```python
from build123d import *

# Parameters (mm, degrees)
SKETCH_1_R          = 4.85
EXTRUDE_1_DEPTH     = 0.5
SKETCH_2_R          = 4
EXTRUDE_2_DEPTH     = 2
SKETCH_3_R          = 3
CUT_EXTRUDE_3_DEPTH = 8.300342458
CHAMFER_1_SIZE      = 0.25


with BuildPart() as part:
    # 草圖1 → 伸長1 (new body)
    with BuildSketch(Plane.XY):
        Circle(SKETCH_1_R)
    extrude(amount=EXTRUDE_1_DEPTH)

    # 草圖2 → 伸長2 (add)
    with BuildSketch(Plane.XY.offset(0.5)):
        Circle(SKETCH_2_R)
    extrude(amount=EXTRUDE_2_DEPTH)

    # 草圖3 → 伸長3 (cut, through all)
    with BuildSketch(Plane.XY.offset(2.5)):
        Circle(SKETCH_3_R)
    extrude(amount=-CUT_EXTRUDE_3_DEPTH, mode=Mode.SUBTRACT)

    # 導角1
    chamfer_1_edges = [part.edges().sort_by_distance(p)[0] for p in [
        (-3, 0, 2.5),
        (-4, 0, 2.5),
    ]]
    chamfer(chamfer_1_edges, length=CHAMFER_1_SIZE)


solid = part.part
```
Verification items for the finished model (mm, model axes). A direction names the side the tool comes from. Round coordinates to 2 decimals unless told otherwise and drop trailing zeros. Loops run counter-clockwise (first coordinate to the right, second up) from the corner with the lowest first, then second, coordinate; pieces in that order, holes last. Notation, with made-up numbers: (75, 29) -> (90, 29) arc R21 ccw to (90, 65) -> close; hole circle Ø11 at (80.25, -22.75). An arc over 180 degrees is marked (long way). Answer as a JSON object with one key per item and string values.
Q1. Access from +Z, -Z, +X, -X, +Y, -Y to the whole of each face (thin tool, end or side, straight path). Record for faces 1 (the flat face through (-1.4, 3.1, 2.5)), 2 (the flat face through (-2, 4, 0.5)).
Data:
{"face 1": "+Z, +X, -X, +Y, -Y", "face 2": "+Z"}
Q2. Section check A-A (y = 0). Record the boundary of the cut face in (x, z), then the cut area to 4 significant figures.
Data:
{"outline": "(-4.85, 0) -> (-3, 0) -> (-3, 2.25) -> (-3.25, 2.5) -> (-3.75, 2.5) -> (-4, 2.25) -> (-4, 0.5) -> (-4.85, 0.5) -> close; (3, 0) -> (4.85, 0) -> (4.85, 0.5) -> (4, 0.5) -> (4, 2.25) -> (3.75, 2.5) -> (3.25, 2.5) -> (3, 2.25) -> close", "area": "5.725 mm2"}
Q3. Draft check along X on faces 3 (the cylindrical face through (-3, 0, 1)), 4 (the flat face through (3.2, 0.1, 0)), 5 (the cylindrical face through (-0.867, -3.905, 1.363)). Enter one of: pulls with the +X half, pulls with the -X half, needs draft (parallel to the pull), parting line crosses it, or undercut.
Data:
{"face 3": "undercut", "face 4": "needs draft", "face 5": "parting line crosses it"}
Q4. Go/stop test with a flat-tipped pin: P1, Ø1.5, axis at y = 1, z = 2, coming from the -X side. Record where the tip stops, or that it passes through.
Data:
{"P1": "stops at x = -3.99"}
Q5. Scan lines: line 1 (Y direction, x = 0, z = 0.9); line 2 (Y direction, x = -0.75, z = 1); line 3 (X direction, y = 1.25, z = 1.1). Record each from-to range of solid material in increasing order. Write a range as from..to.
Data:
{"line 1": "y = -4..-3, 3..4", "line 2": "y = -3.93..-2.9, 2.9..3.93", "line 3": "x = -3.8..-2.73, 2.73..3.8"}
Q6. Section check C-C (z = 2.05). Record the boundary of the cut face in (x, y).
Data:
{"outline": "circle Ø8 at (0, 0); hole circle Ø6 at (0, 0)"}
